Build history of the part. All positions in model axes, mm. Face numbers are marked on the shaded views. A direction names the side the tool comes from. Give positions to 0.01 mm unless a question says otherwise; leave off trailing zeros. Write each loop counter-clockwise with the first axis right and the second up, starting at its lowest first coordinate (ties: lowest second). Pieces come first, ordered by that corner, then holes. Notation, with made-up numbers: (80, -6) -> (101, -6) arc R21 ccw to (101, 20) -> close; hole circle Ø4 at (24.5, 55). An arc over 180 degrees is marked (long way). One line per question, with ' | ' between items. Start each with the question number.
(1) Band-saw the part on D-D, the plane x = -14. Give the cut face in (y, z).
(2) Pin check, flat tips, straight feed: P1, Ø2, axis at x = -11, y = 1.5, coming from the -Z side; P2, Ø12, axis at y = -10, z = 8.5, coming from the +X side; P3, Ø3, axis at y = -17, z = 67.5, coming from the -X side. Stop position of each tip, or through.
(3) Tool access for the marked faces 1, 2 and 3: list every direction of +Z, -Z, +X, -X, +Y, -Y with a clear straight run to the whole face (end or side of a thin tool).
(4) Band-saw the part on A-A, the plane x = 0. Give the cut face in (y, z).
(5) Band-saw the part on C-C, the plane z = 9. Give the cut face in (x, y).
(6) Drill centre lines: probe 1 along Y at (x, z) = (0, 5.5); probe 2 along X at (y, z) = (-0.5, 12) (1 decimal). Where is each one in solid material? Low to high. Write a range as from..to.
from build123d import *

# Parameters (mm, degrees)
F0_R     = 25
F1_DEPTH = 80
F2_R     = 17.5
F3_DEPTH = 11
F4_R     = 17.5
F5_DEPTH = 11
F6_R     = 10
F7_DEPTH = 100


with BuildPart() as f1:
    # F0 (on Top) → F1 (new body)
    with BuildSketch(Plane.XY):
        Circle(F0_R)
    extrude(amount=F1_DEPTH)

    # F2 (on face) → F3 (cut)
    with BuildSketch(Plane.XY.offset(80)):
        Circle(F2_R)
    extrude(amount=-F3_DEPTH, mode=Mode.SUBTRACT)

    # F4 (on face) → F5 (cut)
    with BuildSketch(Plane(origin=(0, 0, 0), x_dir=(1, 0, 0), z_dir=(0, 0, -1))):
        Circle(F4_R)
    extrude(amount=-F5_DEPTH, mode=Mode.SUBTRACT)

    # F6 (on face) → F7 (cut)
    with BuildSketch(Plane(origin=(0, 0, 11), x_dir=(1, 0, 0), z_dir=(0, 0, -1))):
        Circle(F6_R)
    extrude(amount=-F7_DEPTH, mode=Mode.SUBTRACT)


solid = f1.part
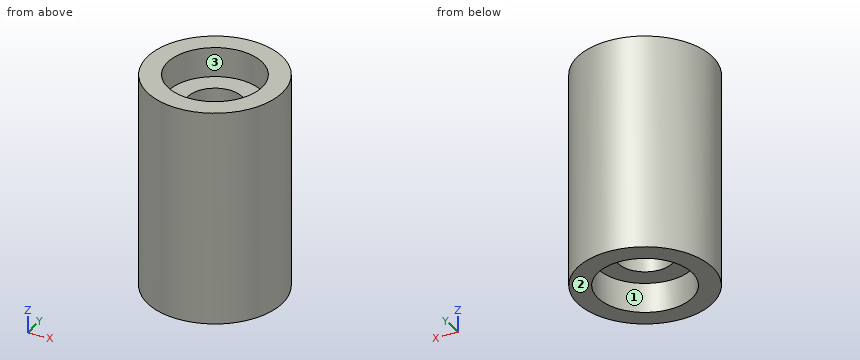
Results:
1) outline: (-20.71, 0) -> (-10.5, 0) -> (-10.5, 11) -> (10.5, 11) -> (10.5, 0) -> (20.71, 0) -> (20.71, 80) -> (10.5, 80) -> (10.5, 69) -> (-10.5, 69) -> (-10.5, 80) -> (-20.71, 80) -> close
2) P1: stops at z = 11 | P2: stops at x = 24.68 | P3: stops at x = -19.62
3) face 1: -Z | face 2: -Z, +X, -X, +Y, -Y | face 3: +Z
4) outline: (-25, 0) -> (-17.5, 0) -> (-17.5, 11) -> (-10, 11) -> (-10, 69) -> (-17.5, 69) -> (-17.5, 80) -> (-25, 80) -> close; (10, 11) -> (17.5, 11) -> (17.5, 0) -> (25, 0) -> (25, 80) -> (17.5, 80) -> (17.5, 69) -> (10, 69) -> close
5) outline: circle Ø50 at (0, 0); hole circle Ø35 at (0, 0)
6) probe 1: y = -25..-17.5, 17.5..25 | probe 2: x = -25..-10, 10..25
